```python
from build123d import *

# Parameters (mm, degrees)
BOSS_EXTRUDE1_DEPTH = 54
CUT_EXTRUDE1_DEPTH  = 1
SKETCH3_R           = 1
CUT_EXTRUDE2_DEPTH  = 55.286278193


with BuildPart() as part:
    # Sketch1 → Boss-Extrude1 (new body)
    with BuildSketch(Plane.XY):
        with BuildLine():
            ThreePointArc((5.361902647, 4.5), (0, 7), (-5.361902647, 4.5))
            Line((-5.361902647, 4.5), (5.361902647, 4.5))
        make_face()
    extrude(amount=BOSS_EXTRUDE1_DEPTH)

    # Sketch2 → Cut-Extrude1 (cut)
    with BuildSketch(Plane.XZ.offset(-4.5)):
        Polygon((2.309401077, 50), (1.154700538, 52), (-1.154700538, 52), (-2.309401077, 50), (-1.154700538, 48), (1.154700538, 48), align=None)
        Polygon((2.309401077, 2), (1.154700538, 4), (-1.154700538, 4), (-2.309401077, 2), (-1.154700538, 0), (1.154700538, 0), align=None)
    extrude(amount=-CUT_EXTRUDE1_DEPTH, mode=Mode.SUBTRACT)

    # Sketch3 → Cut-Extrude2 (cut, through all)
    with BuildSketch(Plane.XZ.offset(-5.5)):
        with Locations(Location((0, 2, 0), (0, 0, 270))):
            Circle(SKETCH3_R)
        with Locations(Location((0, 50, 0), (0, 0, 270))):
            Circle(SKETCH3_R)
    extrude(amount=-CUT_EXTRUDE2_DEPTH, mode=Mode.SUBTRACT)


solid = part.part
```
CAD build for the part. Positions are in the model's coordinates, mm. A direction names the side the tool comes from. Coordinates: 2 decimals unless noted, no trailing zeros. Order: outer loops, then holes, each group sorted by start corner. A loop starts at its lowest first (then second) coordinate and runs counter-clockwise, first axis right, second up.
(1) Saw through at B-B, the plane y = 6.6. Write the cut outline in (x, z).
Solution:
outline: (-2.33, 0) - (2.33, 0) - (2.33, 54) - (-2.33, 54) - close; hole circle Ø2 at (0, 2); hole circle Ø2 at (0, 50)
(2) Which spindle directions (+Z, -Z, +X, -X, +Y, -Y) get a long thin tool onto all of the face, cutting with end or side? Do faces 1 (the face through (-1.724, 4.993, 3.014)), 2 (the face through (0, 5, 4)), 3 (the face through (0, 4.5, 27)). Say none if no direction does.
Solution:
face 1: -Y
face 2: -Z, -Y
face 3: +Z, -Z, +X, -X, -Y
(3) Drill centre lines: L1, parallel to Z at x = 0, y = 6.5; L2, parallel to Z at x = 0.75, y = 4.95; L3, parallel to X at y = 6.15, z = 2. Where is each one in solid material? Low to high.
Solution:
L1: z = 0 to 1, 3 to 49, 51 to 54
L2: z = 4 to 48, 52 to 54
L3: x = -3.34 to -1, 1 to 3.34
(4) Mould opens along X. For faces 4 (the face through (0, 5, 52)), 5 (the face through (0, 5, 54)), 6 (the face through (0, 7, 27)) say: released by +X, released by -X, zero draft, split by the parting line, or undercut.
Solution:
face 4: undercut
face 5: zero draft
face 6: split by the parting line
(5) Saw through at C-C, the plane z = 25.5. Write the cut outline in (x, y).
Solution:
outline: (-5.36, 4.5) - (5.36, 4.5) arc R7 ccw to start
(6) Saw through at D-D, the plane x = 4. Write the cut outline in (y, z), and give its area (3 significant figures).
Solution:
outline: (4.5, 0) - (5.74, 0) - (5.74, 54) - (4.5, 54) - close
area: 67.2 mm2
(7) Pin check, flat tips, straight feed: pin 1 Ø1.5 at (y, z) = (5, 44) entering from -X; pin 2 Ø0.5 at (x, y) = (0, 5) entering from -Z; pin 3 Ø3 at (x, z) = (0, 1.5) entering from -Y; pin 4 Ø1.2 at (x, z) = (0, 2) entering from -Y. Stop position of each tip, or through.
Solution:
pin 1: stops at x = -5.36
pin 2: stops at z = 4
pin 3: stops at y = 5.5
pin 4: passes through
(8) Saw through at A-A, the plane x = 0. Write the cut outline in (y, z).
Solution:
outline: (4.5, 4) - (5.5, 4) - (5.5, 3) - (7, 3) - (7, 49) - (5.5, 49) - (5.5, 48) - (4.5, 48) - close; (4.5, 52) - (5.5, 52) - (5.5, 51) - (7, 51) - (7, 54) - (4.5, 54) - close; (5.5, 0) - (7, 0) - (7, 1) - (5.5, 1) - close
